Input: part model. Units: mm. Frame: model coordinates. Face numbers are marked on the shaded views. Coordinates: 2 decimals unless noted, no trailing zeros. Order: outer loops, then holes, each group sorted by start corner. A loop starts at its lowest first (then second) coordinate and runs counter-clockwise, first axis right, second up. Notation, with made-up numbers: (10, 3.5) -> (66, 3.5) arc R29 ccw to (66, 26.5) -> close; hole circle Ø3 at (0, 1.5). An arc over 180 degrees is marked (long way). Write each question's results on one line, items separated by ' | '.
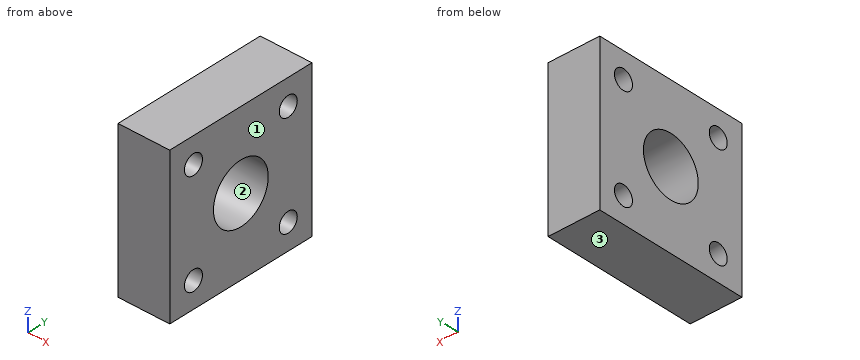
Autodesk Inventor part; units mm, degrees
ref_plane "YZ Plane" through (0, 0, 0) normal (1, 0, 0) x (0, 1, 0)
ref_plane "XZ Plane" through (0, 0, 0) normal (0, 1, 0) x (-1, 0, 0)
ref_plane "XY Plane" through (0, 0, 0) normal (0, 0, 1) x (1, 0, 0)
sketch "Sketch1" plane through (0, 0, 0) normal (1, 0, 0) x (0, 1, 0)
  line L0 (0, -26.67) -> (0, 26.67) construction
  line L1 (-26.67, 0) -> (26.67, 0) construction
  line L2 (19.05, 19.05) -> (-19.05, 19.05)
  line L3 (-19.05, 19.05) -> (-19.05, -19.05)
  line L4 (-19.05, -19.05) -> (19.05, -19.05)
  line L5 (19.05, -19.05) -> (19.05, 19.05)
  circle A0 centre (0, 0) radius 7.3422
  line L6 (12.7, 12.7) -> (-12.7, 12.7) construction
  line L7 (-12.7, 12.7) -> (-12.7, -12.7) construction
  line L8 (-12.7, -12.7) -> (12.7, -12.7) construction
  line L9 (12.7, -12.7) -> (12.7, 12.7) construction
  circle A1 centre (12.7, 12.7) radius 2.413
  circle A2 centre (12.7, -12.7) radius 2.413
  circle A3 centre (-12.7, -12.7) radius 2.413
  circle A4 centre (-12.7, 12.7) radius 2.413
  point P0 (19.05, 0)
  point P1 (0, 19.05)
  point P2 (12.7, 0)
  point P3 (0, 12.7)
  dimension "d0" = 38.1
  dimension "d1" = 14.6844
  dimension "d2" = 4.826
  dimension "d3" = 25.4
extrude "Extrusion1" add sketch "Sketch1" along normal blind 12.7
properties part number "Joint Mount" material "Aluminum 6061"
(1) Cut plane B-B, the plane z = 0. Return loops of the section in (x, y), plus the area to 3 significant figures.
Return value:
outline: (0, -19.05) -> (12.7, -19.05) -> (12.7, -7.34) -> (0, -7.34) -> close; (0, 7.34) -> (12.7, 7.34) -> (12.7, 19.05) -> (0, 19.05) -> close | area: 297 mm2
(2) Line query: line 1 along Z through (x, y) = (6.25, -12.7); line 2 along Z through (x, y) = (5.5, 0); line 3 along Y through (x, z) = (3.5, 10.5). Output: solid intervals per line, ascending. Write a range as from..to.
Return value:
line 1: -19.05..-15.11, -10.29..10.29, 15.11..19.05 | line 2: -19.05..-7.34, 7.34..19.05 | line 3: -19.05..-13.69, -11.71..11.71, 13.69..19.05
(3) Pin query (flat end, axial travel): P1, Ø1, axis at y = 8, z = 14.5, coming from the -X side. Return the tip coordinate at first contact, or that it passes through.
Return value:
P1: x = 0
(4) Mould query, pull axis Z, two halves, no side actions, for the marked faces 1, 2 and 3. Classes: +Z half, -Z half, draft (parallel to the pull), parting line (faces both ways), or undercut.
Return value:
face 1: draft | face 2: undercut | face 3: -Z half
(5) Cut plane D-D, the plane x = 7.25. Return loops of the section in (y, z).
Return value:
outline: (-19.05, -19.05) -> (19.05, -19.05) -> (19.05, 19.05) -> (-19.05, 19.05) -> close; hole circle Ø4.83 at (-12.7, -12.7); hole circle Ø4.83 at (-12.7, 12.7); hole circle Ø14.68 at (0, 0); hole circle Ø4.83 at (12.7, -12.7); hole circle Ø4.83 at (12.7, 12.7)
(6) Cut plane A-A, the plane y = -12.7. Return loops of the section in (x, z), plus the area to 3 significant figures.
Return value:
outline: (0, -19.05) -> (12.7, -19.05) -> (12.7, -15.11) -> (0, -15.11) -> close; (0, -10.29) -> (12.7, -10.29) -> (12.7, 10.29) -> (0, 10.29) -> close; (0, 15.11) -> (12.7, 15.11) -> (12.7, 19.05) -> (0, 19.05) -> close | area: 361 mm2
